Could you check a few things on this drawing? It's one solid part, dimensions in mm from its lowest x, y, z. A direction names the side the tool comes from. Give positions to 0.01 mm unless a question says otherwise; leave off trailing zeros. Loops run counter-clockwise (first coordinate to the right, second up) from the corner with the lowest first, then second, coordinate; pieces in that order, holes last. Notation, with made-up numbers: M 74,71.25 L 117,71.25 A17 cw 117,97.25 Z; hole C -40,63 d11. An arc over 180 degrees is marked long. Return JSON: item names as keys, results as strings. Group by question number.
1. If we section it at A-A (y = 63.5): State how many separate pieces and enclosed holes the cut face has, plus the area to 3 significant figures.
2. For pin 1 (5 mm diameter, centred on y = 12.7, z = 63.5, fed in from +X); pin 2 (2 mm diameter, centred on y = 41, z = 56.5, fed in from +X); pin 3 (6 mm diameter, centred on x = 74.5, y = 57.5, fed in from +Z) (3 decimals), each with a flat end and sliding along its axis, tell me the tip position at first contact or that it passes through.
3. For the marked faces 1 and 2, which set-ups out of +Z, -Z, +X, -X, +Y, -Y let a thin tool reach every point of the face, with its end or its side?
4. Please list where these lines run through material, in increasing order: line 1 (Y direction, x = 2.6, z = 25.4); line 2 (Z direction, x = 1.3, y = 12.7); line 3 (Z direction, x = 2.55, y = 63.5) (1 decimal).
5. If we section it at D-D (z = 41): Write out the boundary of the cut face in (x, y).
6. If we section it at C-C (x = 57): Write out the boundary of the cut face in (y, z) (1 decimal).
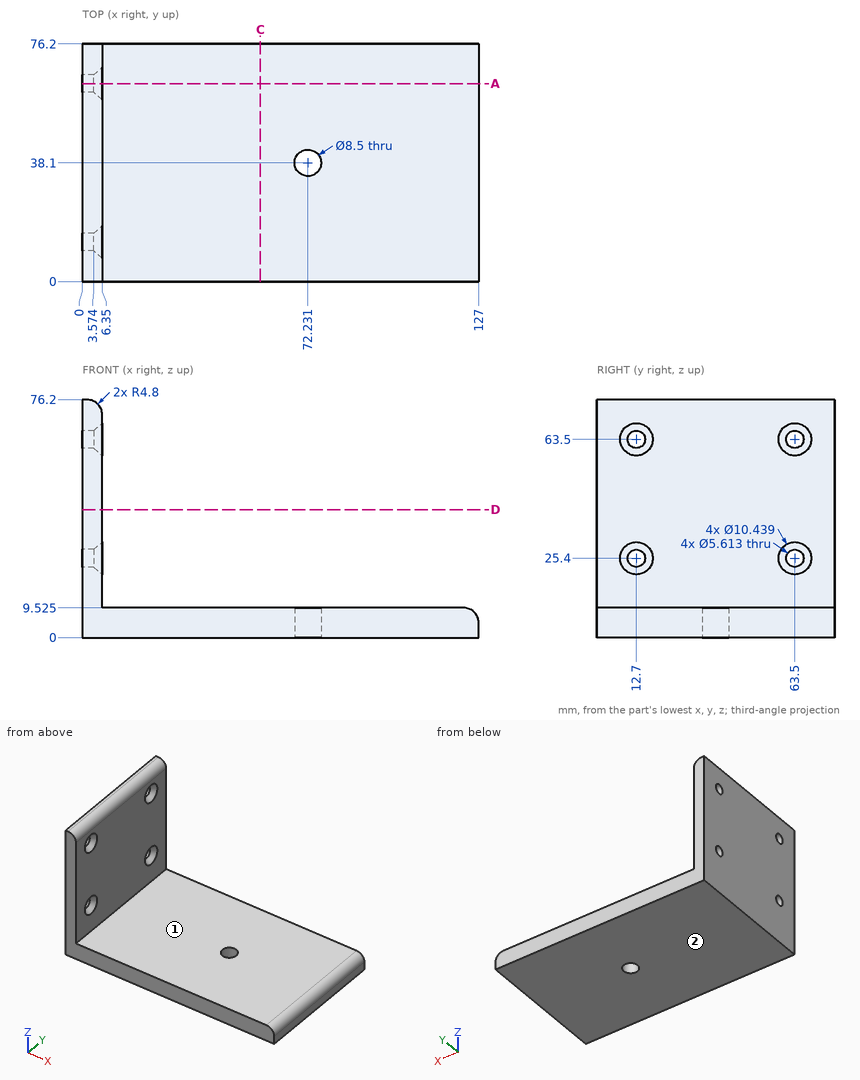
Answer:
{
 "1": {"separate pieces": "3", "enclosed holes": "0", "area": "1,540 mm²"},
 "2": {"pin 1": "passes through", "pin 2": "stops at x = 6.35", "pin 3": "stops at z = 9.525"},
 "3": {"face 1": "+Z, +X, +Y, -Y", "face 2": "-Z, +X, -X, +Y, -Y"},
 "4": {"line 1": "y = 0 to 9.89, 15.51 to 60.69, 66.31 to 76.2", "line 2": "z = 0 to 22.59, 28.21 to 60.69, 66.31 to 76.2", "line 3": "z = 0 to 22.6, 28.2 to 60.7, 66.3 to 76.1"},
 "5": {"outline": "M 0,0 L 6.35,0 L 6.35,76.2 L 0,76.2 Z"},
 "6": {"outline": "M 0,0 L 76.2,0 L 76.2,9.5 L 0,9.5 Z"}
}
